from build123d import *

# Parameters (mm, degrees)
SKETCH_1_W          = 1060
SKETCH_1_H          = 360
EXTRUDE_1_DEPTH     = 20
CUT_EXTRUDE_1_REACH = 562.089
SKETCH_3_R          = 16
SKETCH_3_R_2        = 7
CUT_EXTRUDE_2_DEPTH = 20


with BuildPart() as part:
    # 草图1 → 凸台-拉伸1 (new body)
    with BuildSketch(Plane.XY):
        Rectangle(SKETCH_1_W, SKETCH_1_H)
    extrude(amount=-EXTRUDE_1_DEPTH)

    # 草图2 → 切除-拉伸1 (cut, up to next)
    with BuildSketch(Plane.XY, mode=Mode.PRIVATE) as cut_extrude_1_sk1:
        with BuildLine():
            Line((-530, 180), (-230, 180))
            Line((-230, 180), (-230, 155))
            ThreePointArc((-230, 155), (-238.786796564, 133.786796564), (-260, 125))
            Line((-260, 125), (-530, 125))
            Line((-530, 125), (-530, 180))
        make_face()
    cut_extrude_1_tool1 = extrude(cut_extrude_1_sk1.sketch, amount=-CUT_EXTRUDE_1_REACH, mode=Mode.PRIVATE) & part.part
    # 草图2 → 切除-拉伸1 (cut, up to next)
    with BuildSketch(Plane.XY, mode=Mode.PRIVATE) as cut_extrude_1_sk2:
        with BuildLine():
            Line((230, 180), (230, 155))
            ThreePointArc((230, 155), (238.786796564, 133.786796564), (260, 125))
            Line((260, 125), (530, 125))
            Line((530, 125), (530, 180))
            Line((530, 180), (230, 180))
        make_face()
    cut_extrude_1_tool2 = extrude(cut_extrude_1_sk2.sketch, amount=-CUT_EXTRUDE_1_REACH, mode=Mode.PRIVATE) & part.part
    # 草图2 → 切除-拉伸1 (cut, up to next)
    with BuildSketch(Plane.XY, mode=Mode.PRIVATE) as cut_extrude_1_sk3:
        with BuildLine():
            Line((530, -180), (230, -180))
            Line((230, -180), (230, -155))
            ThreePointArc((230, -155), (238.786796564, -133.786796564), (260, -125))
            Line((260, -125), (530, -125))
            Line((530, -125), (530, -180))
        make_face()
    cut_extrude_1_tool3 = extrude(cut_extrude_1_sk3.sketch, amount=-CUT_EXTRUDE_1_REACH, mode=Mode.PRIVATE) & part.part
    # 草图2 → 切除-拉伸1 (cut, up to next)
    with BuildSketch(Plane.XY, mode=Mode.PRIVATE) as cut_extrude_1_sk4:
        with BuildLine():
            Line((-230, -180), (-230, -155))
            ThreePointArc((-230, -155), (-238.786796564, -133.786796564), (-260, -125))
            Line((-260, -125), (-530, -125))
            Line((-530, -125), (-530, -180))
            Line((-530, -180), (-230, -180))
        make_face()
    cut_extrude_1_tool4 = extrude(cut_extrude_1_sk4.sketch, amount=-CUT_EXTRUDE_1_REACH, mode=Mode.PRIVATE) & part.part
    add(cut_extrude_1_tool1.solids().sort_by_distance((-381.697261, 152.746347, 0))[0], mode=Mode.SUBTRACT)
    add(cut_extrude_1_tool2.solids().sort_by_distance((381.697261, 152.746347, 0))[0], mode=Mode.SUBTRACT)
    add(cut_extrude_1_tool3.solids().sort_by_distance((381.697261, -152.746347, 0))[0], mode=Mode.SUBTRACT)
    add(cut_extrude_1_tool4.solids().sort_by_distance((-381.697261, -152.746347, 0))[0], mode=Mode.SUBTRACT)

    # 草图3 → 切除-拉伸2 (cut)
    with BuildSketch(Plane.XY):
        with Locations((-195, 155)):
            Circle(SKETCH_3_R)
        with Locations((-65, 155)):
            Circle(SKETCH_3_R)
        with Locations((65, 155)):
            Circle(SKETCH_3_R)
        with Locations((195, 155)):
            Circle(SKETCH_3_R)
        with Locations((195, -155)):
            Circle(SKETCH_3_R)
        with Locations((65, -155)):
            Circle(SKETCH_3_R)
        with Locations((-65, -155)):
            Circle(SKETCH_3_R)
        with Locations((-195, -155)):
            Circle(SKETCH_3_R)
        with Locations((-500, 95)):
            Circle(SKETCH_3_R_2)
        with Locations((-430, 95)):
            Circle(SKETCH_3_R_2)
        with Locations((-360, 95)):
            Circle(SKETCH_3_R_2)
        with Locations((-500, 35)):
            Circle(SKETCH_3_R_2)
        with Locations((-500, -35)):
            Circle(SKETCH_3_R_2)
        with Locations((-500, -95)):
            Circle(SKETCH_3_R_2)
        with Locations((-360, 35)):
            Circle(SKETCH_3_R_2)
        with Locations((-360, -35)):
            Circle(SKETCH_3_R_2)
        with Locations((-360, -95)):
            Circle(SKETCH_3_R_2)
        with Locations((-430, -95)):
            Circle(SKETCH_3_R_2)
        with Locations((430, -95)):
            Circle(SKETCH_3_R_2)
        with Locations((360, -95)):
            Circle(SKETCH_3_R_2)
        with Locations((360, -35)):
            Circle(SKETCH_3_R_2)
        with Locations((360, 35)):
            Circle(SKETCH_3_R_2)
        with Locations((500, -95)):
            Circle(SKETCH_3_R_2)
        with Locations((500, -35)):
            Circle(SKETCH_3_R_2)
        with Locations((500, 35)):
            Circle(SKETCH_3_R_2)
        with Locations((360, 95)):
            Circle(SKETCH_3_R_2)
        with Locations((430, 95)):
            Circle(SKETCH_3_R_2)
        with Locations((500, 95)):
            Circle(SKETCH_3_R_2)
        with BuildLine():
            Line((-471, 76), (-389, 76))
            ThreePointArc((-389, 76), (-381.928932188, 73.071067812), (-379, 66))
            Line((-379, 66), (-379, -66))
            ThreePointArc((-379, -66), (-381.928932188, -73.071067812), (-389, -76))
            Line((-389, -76), (-471, -76))
            ThreePointArc((-471, -76), (-478.071067812, -73.071067812), (-481, -66))
            Line((-481, -66), (-481, 66))
            ThreePointArc((-481, 66), (-478.071067812, 73.071067812), (-471, 76))
        make_face()
        with BuildLine():
            Line((379, 66), (379, -66))
            ThreePointArc((379, -66), (381.928932188, -73.071067812), (389, -76))
            Line((389, -76), (471, -76))
            ThreePointArc((471, -76), (478.071067812, -73.071067812), (481, -66))
            Line((481, -66), (481, 66))
            ThreePointArc((481, 66), (478.071067812, 73.071067812), (471, 76))
            Line((471, 76), (389, 76))
            ThreePointArc((389, 76), (381.928932188, 73.071067812), (379, 66))
        make_face()
    extrude(amount=-CUT_EXTRUDE_2_DEPTH, mode=Mode.SUBTRACT)


solid = part.part
For this review, take the finished solid that the model builds, in its own axes (mm). A direction names the side the tool comes from. Coordinates: 2 decimals unless noted, no trailing zeros. Loops run counter-clockwise (first coordinate to the right, second up) from the corner with the lowest first, then second, coordinate; pieces in that order, holes last. Notation, with made-up numbers: (14, 68.25) - (69, 68.25) arc R11 ccw to (69, 84.25) - close; hole circle Ø3 at (85.25, 14). An arc over 180 degrees is marked (long way). Return JSON: item names as keys, results as strings.
Item 1: Take a section at D-D (x = -342.5). Give the boundary of the cut face in (y, z).
Determined:
{"outline": "(-125, -20) - (125, -20) - (125, 0) - (-125, 0) - close"}
Item 2: Insertion check: pin 1 (10 mm diameter, centred on x = 378, z = -9.5, fed in from -Y); pin 2 (6 mm diameter, centred on x = -401.5, z = -11.5, fed in from +Y); pin 3 (10 mm diameter, centred on y = 172, z = -9, fed in from -X). Each pin has a flat end and moves straight along its axis. Give the tip position at first contact, or say it passes through.
Determined:
{"pin 1": "stops at y = -125", "pin 2": "stops at y = 125", "pin 3": "stops at x = -230"}
Item 3: Take a section at A-A (y = -13). Give the boundary of the cut face in (x, z).
Determined:
{"outline": "(-530, -20) - (-481, -20) - (-481, 0) - (-530, 0) - close; (-379, -20) - (379, -20) - (379, 0) - (-379, 0) - close; (481, -20) - (530, -20) - (530, 0) - (481, 0) - close"}
Item 4: Take a section at B-B (x = -65). Give the boundary of the cut face in (y, z).
Determined:
{"outline": "(-180, -20) - (-171, -20) - (-171, 0) - (-180, 0) - close; (-139, -20) - (139, -20) - (139, 0) - (-139, 0) - close; (171, -20) - (180, -20) - (180, 0) - (171, 0) - close"}
Item 5: For line 1 (Y direction, x = 500, z = -11); line 2 (X direction, y = 9, z = -7); line 3 (Y direction, x = 193, z = -12.5), list the stretches that pass through material, from the lowest coordinate up.
Determined:
{"line 1": "y = -125 to -102, -88 to -42, -28 to 28, 42 to 88, 102 to 125", "line 2": "x = -530 to -481, -379 to 379, 481 to 530", "line 3": "y = -180 to -170.87, -139.13 to 139.13, 170.87 to 180"}
Item 6: Take a section at C-C (z = -6.5). State how many separate pieces and enclosed holes the cut face has, then the cut area to 3 significant figures.
Determined:
{"separate pieces": "1", "enclosed holes": "30", "area": "276,000 mm2"}
Item 7: Mouldability with a two-part tool opening along Y and no side actions: class faces 1 (the cylindrical face through (-67.083, -139.136, -9.86)), 2 (the flat face through (-3, -180, -10)), 3 (the flat face through (-3, 180, -10)), 4 (the flat face through (-230, 168, -10)) as pulls with the +Y half, pulls with the -Y half, needs draft (parallel to the pull), parting line crosses it, or undercut.
Determined:
{"face 1": "undercut", "face 2": "pulls with the -Y half", "face 3": "pulls with the +Y half", "face 4": "needs draft"}
Item 8: For faces 5 (the cylindrical face through (238.555, -134.021, -9.86)), 6 (the flat face through (-230, -168, -10)), 7 (the flat face through (431, 76, -10)), list the 3-axis set-ups (+Z, -Z, +X, -X, +Y, -Y) from which the entire face can be reached by the end or side of a thin tool; tool diameter is ignored.
Determined:
{"face 5": "+Z, -Z, +X, -Y", "face 6": "+Z, -Z, -X, -Y", "face 7": "+Z, -Z"}
